Work out the finished part from the listing and answer in its coordinate system (mm). Give positions to 0.01 mm unless a question says otherwise; leave off trailing zeros. Order: outer loops, then holes, each group sorted by start corner. A loop starts at its lowest first (then second) coordinate and runs counter-clockwise, first axis right, second up. Notation, with made-up numbers: (12.25, -8) - (24.25, -8) arc R26 ccw to (24.25, 20) - close; hole circle Ø2 at (-10.75, 73.5). An arc over 180 degrees is marked (long way). Put each result on its own line as item: value.
```python
from build123d import *

# Parameters (mm, degrees)
EXTRUDE1_DEPTH      = 3.96875
EXTRUDE1_DEPTH_BACK = 3.96875
SKETCH1_R           = 3.175
SKETCH1_R_2         = 1.4224
SKETCH13_OUTSIDE_W  = 10.748
SKETCH13_OUTSIDE_H  = 10.748
SKETCH13_OUTSIDE_R  = 2.38125
CUT_EXTRUDE1_DEPTH  = 10.119493201


with BuildPart() as part:
    # Sketch1 → Extrude1 (new, two sides: drawn at the far end of the back side and taken through both)
    with BuildSketch(Plane.XY.offset(-EXTRUDE1_DEPTH_BACK)):
        Circle(SKETCH1_R)
        Circle(SKETCH1_R_2, mode=Mode.SUBTRACT)
    extrude(amount=EXTRUDE1_DEPTH + EXTRUDE1_DEPTH_BACK)

    # Extrude3 cone 1 section (through the dimple's axis) → Extrude3 (revolve, cut)
    with BuildSketch(Plane(origin=(0, 0, -3.96875), x_dir=(0, 1, 0), z_dir=(1, 0, 0))):
        Polygon((0, 0), (1.4732, 0), (0, 1.579813584), align=None)
    extrude3 = revolve(axis=Axis((0, 0, -3.96875), (0, 0, 1)), mode=Mode.SUBTRACT)

    # Mirror1: Extrude3 across plane
    add(extrude3.mirror(Plane.XY), mode=Mode.SUBTRACT)

    # Sketch13 outside → Cut-Extrude1 (cut, through all)
    with BuildSketch(Plane.XY.offset(3.96875)):
        Rectangle(SKETCH13_OUTSIDE_W, SKETCH13_OUTSIDE_H)
        Circle(SKETCH13_OUTSIDE_R, mode=Mode.SUBTRACT)
    extrude(amount=-CUT_EXTRUDE1_DEPTH, mode=Mode.SUBTRACT)


solid = part.part
```
(1) Given pin 1 (1.7 mm diameter, centred on x = 0, y = 0, fed in from +Z); pin 2 (1 mm diameter, centred on y = -1.5, z = -0.5, fed in from +X); pin 3 (1.5 mm diameter, centred on y = -2, z = -3, fed in from +X), each flat-ended and moving along its own axis, determine where each tip first touches the part or whether it passes through.
Geometry check:
pin 1: passes through
pin 2: stops at x = 2.16
pin 3: stops at x = 2.03
(2) Determine the mould class of faces 1 (the face through (0, -2, -3.969)), 2 (the face through (-1.89, -1.45, 0.06)), 3 (the face through (-0.31, -1.39, -0.05)) for opening direction X: pulls with the +X half, pulls with the -X half, needs draft (parallel to the pull), parting line crosses it, or undercut.
Geometry check:
face 1: needs draft
face 2: parting line crosses it
face 3: undercut
(3) Section D-D, the plane y = 1.95 is taken. Write down the section's boundary in (x, z), then the cut area to 3 significant figures.
Geometry check:
outline: (-1.37, -3.97) - (1.37, -3.97) - (1.37, 3.97) - (-1.37, 3.97) - close
area: 21.7 mm²
(4) Straight lines are drawn through the part: line 1 (Y direction, x = 0, z = 0.5); line 2 (Y direction, x = 0.55, z = -2); line 3 (X direction, y = -0.2, z = -0.25). For each, find the intervals that lie inside material, in ascending order.
Geometry check:
line 1: y = -2.38 to -1.42, 1.42 to 2.38
line 2: y = -2.32 to -1.31, 1.31 to 2.32
line 3: x = -2.37 to -1.41, 1.41 to 2.37
(5) Section A-A, the plane x = 0 is taken. Write down the section's boundary in (y, z).
Geometry check:
outline: (-2.38, -3.97) - (-1.47, -3.97) - (-1.42, -3.91) - (-1.42, 3.91) - (-1.47, 3.97) - (-2.38, 3.97) - close; (1.42, -3.91) - (1.47, -3.97) - (2.38, -3.97) - (2.38, 3.97) - (1.47, 3.97) - (1.42, 3.91) - close
(6) Section C-C, the plane z = -1 is taken. Write down the section's boundary in (x, y).
Geometry check:
outline: circle Ø4.76 at (0, 0); hole circle Ø2.84 at (0, 0)
